```python
from build123d import *

# Parameters (mm, degrees)
F0_R     = 9.95
F0_R_2   = 11
F1_DEPTH = 5


with BuildPart() as f1:
    # F0 (on Top) → F1 (new body)
    with BuildSketch(Plane.XY):
        with BuildLine():
            ThreePointArc((8.291562, -12.5), (15, 0), (8.291562, 12.5))
            ThreePointArc((8.291562, 12.5), (0, 40), (-8.291562, 12.5))
            ThreePointArc((-8.291562, 12.5), (-15, 0), (-8.291562, -12.5))
            ThreePointArc((-8.291562, -12.5), (0, -40), (8.291562, -12.5))
        make_face()
        with Locations((0, -25)):
            Circle(F0_R, mode=Mode.SUBTRACT)
        Circle(F0_R_2, mode=Mode.SUBTRACT)
        with Locations((0, 25)):
            Circle(F0_R, mode=Mode.SUBTRACT)
    extrude(amount=F1_DEPTH)


solid = f1.part
```
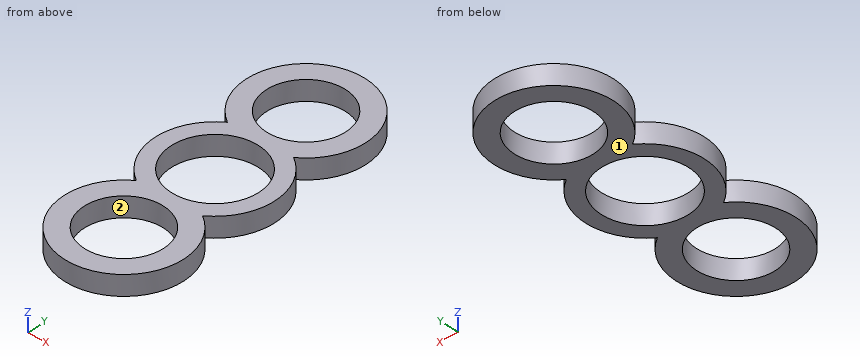
Here's how the part is built. I have some questions about the finished solid (model axes, mm). Face numbers are marked on the shaded views. Give positions to 0.01 mm unless a question says otherwise; leave off trailing zeros. Write each loop counter-clockwise with the first axis right and the second up, starting at its lowest first coordinate (ties: lowest second). Pieces come first, ordered by that corner, then holes. Notation, with made-up numbers: (54.5, 14.25) -> (73.5, 14.25) arc R8 cw to (73.5, 28.25) -> close; hole circle Ø4 at (-23, 33.5). An arc over 180 degrees is marked (long way). Use one line per item in the form item = value.
1) Suppose I cut it at D-D (x = 9). Please give me the cut outline in (y, z), and give its area (3 significant figures).
Verdict:
outline = (-37, 0) -> (-29.24, 0) -> (-29.24, 5) -> (-37, 5) -> close; (-20.76, 0) -> (-13, 0) -> (-13, 5) -> (-20.76, 5) -> close; (-12, 0) -> (-6.32, 0) -> (-6.32, 5) -> (-12, 5) -> close; (6.32, 0) -> (12, 0) -> (12, 5) -> (6.32, 5) -> close; (13, 0) -> (20.76, 0) -> (20.76, 5) -> (13, 5) -> close; (29.24, 0) -> (37, 0) -> (37, 5) -> (29.24, 5) -> close
area = 212 mm2
2) If I drill on L1, parallel to Y at x = 0, z = 3.1; L2, parallel to Y at x = -6, z = 4.05; L3, parallel to Y at x = -9, z = 3.55, over which ranges is the centre line in solid material (lowest first)? Write a range as [from, to].
Verdict:
L1 = [-40, -34.95], [-15.05, -11], [11, 15.05], [34.95, 40]
L2 = [-38.75, -32.94], [-17.06, -9.22], [9.22, 17.06], [32.94, 38.75]
L3 = [-37, -29.24], [-20.76, -13], [-12, -6.32], [6.32, 12], [13, 20.76], [29.24, 37]
3) Suppose I cut it at B-B (x = 0). Please give me the cut outline in (y, z), and give its area (3 significant figures).
Verdict:
outline = (-40, 0) -> (-34.95, 0) -> (-34.95, 5) -> (-40, 5) -> close; (-15.05, 0) -> (-11, 0) -> (-11, 5) -> (-15.05, 5) -> close; (11, 0) -> (15.05, 0) -> (15.05, 5) -> (11, 5) -> close; (34.95, 0) -> (40, 0) -> (40, 5) -> (34.95, 5) -> close
area = 91.0 mm2
4) Suppose I cut it at C-C (z = 3.85). Please give me the cut outline in (x, y), and give its area (3 significant figures).
Verdict:
outline = (-8.29, -12.5) arc R15 ccw (long way) to (8.29, -12.5) arc R15 ccw to (8.29, 12.5) arc R15 ccw (long way) to (-8.29, 12.5) arc R15 ccw to start; hole circle Ø22 at (0, 0); hole circle Ø19.9 at (0, -25); hole circle Ø19.9 at (0, 25)
area = 1,010 mm2
5) I'm going to push flat-ended pins straight in: pin 1 (1 mm diameter, centred on y = 26, z = 1, fed in from +X); pin 2 (1.5 mm diameter, centred on x = 11.5, z = 3, fed in from +Y). Where does each tip first touch, or does it pass through?
Verdict:
pin_1 = 14.99
pin_2 = 35.46
6) We'd pull the mould along Y, two halves only. Please class the marked faces 1 and 2: +Y half, -Y half, draft (parallel to the pull), parting line (faces both ways), or undercut.
Verdict:
face_1 = draft
face_2 = undercut
7) Suppose I cut it at A-A (y = 0). Please give me the cut outline in (x, z), and give its area (3 significant figures).
Verdict:
outline = (-15, 0) -> (-11, 0) -> (-11, 5) -> (-15, 5) -> close; (11, 0) -> (15, 0) -> (15, 5) -> (11, 5) -> close
area = 40.0 mm2
